Here's how the part is built. I have some questions about the finished solid (model axes, mm). A direction names the side the tool comes from. Coordinates: 2 decimals unless noted, no trailing zeros. Order: outer loops, then holes, each group sorted by start corner. A loop starts at its lowest first (then second) coordinate and runs counter-clockwise, first axis right, second up. Notation, with made-up numbers: (-25, 33) - (-9, 33) arc R27 ccw to (-9, 52) - close; hole circle Ø9 at (88, 79.25). An arc over 180 degrees is marked (long way). Use CSV: the item, a comma, the result in double quotes. Start each with the question number.
from build123d import *

# Parameters (mm, degrees)
F0_R     = 9.6
F1_DEPTH = 10
F3_R     = 11.125
F4_DEPTH = 2
F5_SIZE  = 1
F6_R     = 3.175
F7_DEPTH = 12.001
F9_DEPTH = 0.5


with BuildPart() as f1:
    # F0 (on Top) → F1 (new body)
    with BuildSketch(Plane.XY):
        Circle(F0_R)
    extrude(amount=-F1_DEPTH)

    # F3 (on face) → F4 (join)
    with BuildSketch(Plane.XY):
        Circle(F3_R)
    extrude(amount=F4_DEPTH)

    # F5
    f5_edges = [f1.edges().sort_by_distance(p)[0] for p in [
        (-11.125, 0, 2),
    ]]
    chamfer(f5_edges, length=F5_SIZE)

    # F6 (on face) → F7 (cut, through all)
    with BuildSketch(Plane.XY.offset(2)):
        Circle(F6_R)
    extrude(amount=-F7_DEPTH, mode=Mode.SUBTRACT)

    # F8 (on face) → F9 (cut)
    with BuildSketch(Plane.XY.offset(2)):
        Polygon((1.5, 5.125), (0, 9.125), (-1.5, 5.125), align=None)
    extrude(amount=-F9_DEPTH, mode=Mode.SUBTRACT)


solid = f1.part
Item 1: For pin 1 Ø4 at (x, z) = (-1, -6) entering from +Y; pin 2 Ø3 at (y, z) = (7.5, -7.5) entering from +X; pin 3 Ø6 at (x, z) = (5, -4) entering from -Y, each with a flat end and sliding along its axis, tell me the tip position at first contact or that it passes through.
Item 2: We'd pull the mould along X, two halves only. Please class faces 1 (the flat face through (-10, 0, 0)), 2 (the cylindrical face through (-8.2, 7.52, 0.49)), 3 (the flat face through (0, 7, 1.5)): released by +X, released by -X, zero draft, split by the parting line, or undercut.
Item 3: Suppose I cut it at A-A on y = 0. Write out the boundary of the cut face in (x, z) (3 decimals).
Item 4: Suppose I cut it at B-B on z = -4.5. Write out the boundary of the cut face in (x, y) (3 decimals).
Item 5: Please list where these lines run through material, in increasing order: line 1 along Y through (x, z) = (0, -2) (3 decimals); line 2 along Y through (x, z) = (-1, -8.75); line 3 along X through (y, z) = (-1.75, -6.5). Write a range as from..to.
Item 6: For faces 4 (the cylindrical face through (-0.69, -3.1, -3.92)), 5 (the flat face through (0.76, 7.1, 1.75)), 6 (the cylindrical face through (5.161, 8.095, -4.93)), which set-ups out of +Z, -Z, +X, -X, +Y, -Y let a thin tool reach every point of the face, with its end or its side?
Here are the results:
1,pin 1,"y = 9.6"
1,pin 2,"x = 7.49"
1,pin 3,"y = -9.39"
2,face 1,"zero draft"
2,face 2,"split by the parting line"
2,face 3,"undercut"
3,outline,"(-11.125, 0) - (-9.6, 0) - (-9.6, -10) - (-3.175, -10) - (-3.175, 2) - (-10.125, 2) - (-11.125, 1) - close; (3.175, -10) - (9.6, -10) - (9.6, 0) - (11.125, 0) - (11.125, 1) - (10.125, 2) - (3.175, 2) - close"
4,outline,"circle Ø19.2 at (0, 0); hole circle Ø6.35 at (0, 0)"
5,line 1,"-9.6..-3.175, 3.175..9.6"
5,line 2,"-9.55..-3.01, 3.01..9.55"
5,line 3,"-9.44..-2.65, 2.65..9.44"
6,face 4,"+Z, -Z"
6,face 5,"+Z"
6,face 6,"-Z"
